For this review, take the finished solid that the model builds, in its own axes (mm). A direction names the side the tool comes from. Coordinates: 2 decimals unless noted, no trailing zeros. Order: outer loops, then holes, each group sorted by start corner. A loop starts at its lowest first (then second) coordinate and runs counter-clockwise, first axis right, second up. Notation, with made-up numbers: M 8.5,41.5 L 26.5,41.5 A19 cw 26.5,60.5 Z; hole C 39,89.25 d4. An arc over 180 degrees is marked long. Use CSV: the item, a comma, the result in double quotes.
```python
from build123d import *

# Parameters (mm, degrees)
SM_BASE_FLANGE_1_DEPTH = 332.5
SKETCH_6_R             = 5.25
SKETCH_6_R_2           = 2.5
CUT_EXTRUDE_1_DEPTH    = 10
CUT_EXTRUDE_2_DEPTH    = 10


# Sheet-metal steps are written as plain solids
with BuildPart() as part:
    # Sketch 1 → Базовая кромка1 (new, symmetric)
    with BuildSketch(Plane.XY):
        with BuildLine():
            Line((-28, 49), (-28, 27))
            ThreePointArc((-28, 27), (-26.828427125, 24.171572875), (-24, 23))
            Line((-24, 23), (-2, 23))
            ThreePointArc((-2, 23), (-0.585786438, 22.414213562), (0, 21))
            Line((0, 21), (0, -21))
            ThreePointArc((0, -21), (-0.585786438, -22.414213562), (-2, -23))
            Line((-2, -23), (-24, -23))
            ThreePointArc((-24, -23), (-26.828427125, -24.171572875), (-28, -27))
            Line((-28, -27), (-28, -49))
            Line((-28, -49), (-26, -49))
            Line((-26, -49), (-26, -27))
            ThreePointArc((-26, -27), (-25.414213562, -25.585786438), (-24, -25))
            Line((-24, -25), (-2, -25))
            ThreePointArc((-2, -25), (0.828427125, -23.828427125), (2, -21))
            Line((2, -21), (2, 21))
            ThreePointArc((2, 21), (0.828427125, 23.828427125), (-2, 25))
            Line((-2, 25), (-24, 25))
            ThreePointArc((-24, 25), (-25.414213562, 25.585786438), (-26, 27))
            Line((-26, 27), (-26, 49))
            Line((-26, 49), (-28, 49))
        make_face()
    extrude(amount=SM_BASE_FLANGE_1_DEPTH, both=True)

    # Эскиз6 → Вырез-Вытянуть1 (cut)
    with BuildSketch(Plane(origin=(-26, 0, 0), x_dir=(0, 0, -1), z_dir=(1, 0, 0))):
        with Locations(Location((290, 40, 0), (0, 0, 90))):
            Circle(SKETCH_6_R)
        with Locations(Location((265, 40, 0), (0, 0, 90))):
            Circle(SKETCH_6_R)
        with Locations(Location((205, 42.5, 0), (0, 0, 90))):
            Circle(SKETCH_6_R_2)
        with Locations(Location((115, 42.5, 0), (0, 0, 90))):
            Circle(SKETCH_6_R_2)
        with Locations(Location((25, 42.5, 0), (0, 0, 90))):
            Circle(SKETCH_6_R_2)
        with Locations(Location((-115, 42.5, 0), (0, 0, 270))):
            Circle(SKETCH_6_R_2)
        with Locations(Location((-205, 42.5, 0), (0, 0, 270))):
            Circle(SKETCH_6_R_2)
        with Locations(Location((-265, 40, 0), (0, 0, 270))):
            Circle(SKETCH_6_R)
        with Locations(Location((-290, 40, 0), (0, 0, 270))):
            Circle(SKETCH_6_R)
    cut_extrude_1 = extrude(amount=-CUT_EXTRUDE_1_DEPTH, mode=Mode.SUBTRACT)

    # Зеркальное отражение1: Вырез-Вытянуть1 across plane
    add(cut_extrude_1.mirror(Plane.ZX), mode=Mode.SUBTRACT)

    # Эскиз7 → Вырез-Вытянуть2 (cut)
    with BuildSketch(Plane(origin=(2, 0, 0), x_dir=(0, 0, -1), z_dir=(1, 0, 0))):
        with BuildLine():
            Line((-316, 6.5), (-289, 6.5))
            ThreePointArc((-289, 6.5), (-282.5, 0), (-289, -6.5))
            Line((-289, -6.5), (-316, -6.5))
            ThreePointArc((-316, -6.5), (-322.5, 0), (-316, 6.5))
        make_face()
        with BuildLine():
            Line((-233.5, 6.5), (-206.5, 6.5))
            ThreePointArc((-206.5, 6.5), (-200, 0), (-206.5, -6.5))
            Line((-206.5, -6.5), (-233.5, -6.5))
            ThreePointArc((-233.5, -6.5), (-240, 0), (-233.5, 6.5))
        make_face()
        with BuildLine():
            Line((-13.5, 6.5), (13.5, 6.5))
            ThreePointArc((13.5, 6.5), (20, 0), (13.5, -6.5))
            Line((13.5, -6.5), (-13.5, -6.5))
            ThreePointArc((-13.5, -6.5), (-20, 0), (-13.5, 6.5))
        make_face()
        with BuildLine():
            Line((316, 6.5), (289, 6.5))
            ThreePointArc((289, 6.5), (282.5, 0), (289, -6.5))
            Line((289, -6.5), (316, -6.5))
            ThreePointArc((316, -6.5), (322.5, 0), (316, 6.5))
        make_face()
        with BuildLine():
            Line((233.5, 6.5), (206.5, 6.5))
            ThreePointArc((206.5, 6.5), (200, 0), (206.5, -6.5))
            Line((206.5, -6.5), (233.5, -6.5))
            ThreePointArc((233.5, -6.5), (240, 0), (233.5, 6.5))
        make_face()
    extrude(amount=-CUT_EXTRUDE_2_DEPTH, mode=Mode.SUBTRACT)


solid = part.part
```
Item 1: To check wall thickness, follow line 1 along Y through (x, z) = (-26.8, -205); line 2 along Y through (x, z) = (-2, -235); line 3 along Y through (x, z) = (-27.35, -205). State the ranges of each line that lie inside material, in increasing order. Write a range as [from, to].
Solutions:
line 1,"[-49, -45], [-40, -24.14], [24.14, 40], [45, 49]"
line 2,"[-25, -23], [23, 25]"
line 3,"[-49, -45], [-40, -24.81], [24.81, 40], [45, 49]"
Item 2: Clearance check with flat-ended pins moving along their axes: pin 1 Ø1 at (x, z) = (1, -224.5) entering from +Y; pin 2 Ø0.6 at (x, z) = (0.5, 304) entering from -Y; pin 3 Ø0.6 at (x, z) = (1, -307) entering from -Y. State where each tip first meets the part, or that it passes through.
Solutions:
pin 1,"y = 24.12"
pin 2,"y = -24.34"
pin 3,"y = -23.95"
Item 3: Draft analysis for pull direction Y (two halves, no side actions). For faces 1 (the face through (-13, 23, 5)), 2 (the face through (0.3, 0.2, -332.5)), 3 (the face through (-13, 25, 5)), state which applies: released by +Y, released by -Y, zero draft, split by the parting line, or undercut.
Solutions:
face 1,"undercut"
face 2,"zero draft"
face 3,"released by +Y"
Item 4: For faces 4 (the face through (-26, -38, 5)), 5 (the face through (-13, -23, 5)), 6 (the face through (-26, 38, 5)), list the 3-axis set-ups (+Z, -Z, +X, -X, +Y, -Y) from which the entire face can be reached by the end or side of a thin tool; tool diameter is ignored.
Solutions:
face 4,"+Z, -Z, +X, -Y"
face 5,"+Z, -Z, -X"
face 6,"+Z, -Z, +X, +Y"
Item 5: Add section A-A on x = -11. State the section outline as (y, z) points, and give its area (3 significant figures).
Solutions:
outline,"M -25,-332.5 L -23,-332.5 L -23,332.5 L -25,332.5 Z; M 23,-332.5 L 25,-332.5 L 25,332.5 L 23,332.5 Z"
area,"2,660 mm^2"
